Build history of the part. All positions in model axes, mm. Face numbers are marked on the shaded views. A direction names the side the tool comes from. Round coordinates to 2 decimals unless told otherwise and drop trailing zeros. Loops run counter-clockwise (first coordinate to the right, second up) from the corner with the lowest first, then second, coordinate; pieces in that order, holes last. Notation, with made-up numbers: M -28,-37 L -22,-37 A20 cw -22,-29 Z; hole C 69,35 d5. An arc over 180 degrees is marked long. Write each question's results on one line, items separated by ' | '. Start each with the question number.
```python
from build123d import *

# Parameters (mm, degrees)
BOSS_EXTRUDE1_DEPTH = 1.366666667
BOSS_EXTRUDE2_DEPTH = 8.2
FILLET1_R           = 0.5


with BuildPart() as part:
    # Sketch1 → Boss-Extrude1 (new body)
    with BuildSketch(Plane.XY):
        with BuildLine():
            Line((-33.5, 20), (-33.5, -20))
            ThreePointArc((-33.5, -20), (0, -17.434472888), (33.5, -20))
            Line((33.5, -20), (33.5, 20))
            Line((33.5, 20), (-33.5, 20))
        make_face()
    extrude(amount=BOSS_EXTRUDE1_DEPTH)

    # Sketch2 → Boss-Extrude2 (add)
    with BuildSketch(Plane.XY.offset(1.366666667)):
        with BuildLine():
            Line((32.5, -15), (-32.5, -15))
            Line((-32.5, -15), (-32.5, 15))
            ThreePointArc((-32.5, 15), (0, 17.727407049), (32.5, 15))
            Line((32.5, 15), (32.5, -15))
        make_face()
    extrude(amount=BOSS_EXTRUDE2_DEPTH)

    # Fillet1
    fillet1_edges = [part.edges().sort_by_distance(p)[0] for p in [
        (33.5, 0, 1.366666667),
        (-33.5, 0, 1.366666667),
    ]]
    fillet(fillet1_edges, radius=FILLET1_R)


solid = part.part
```
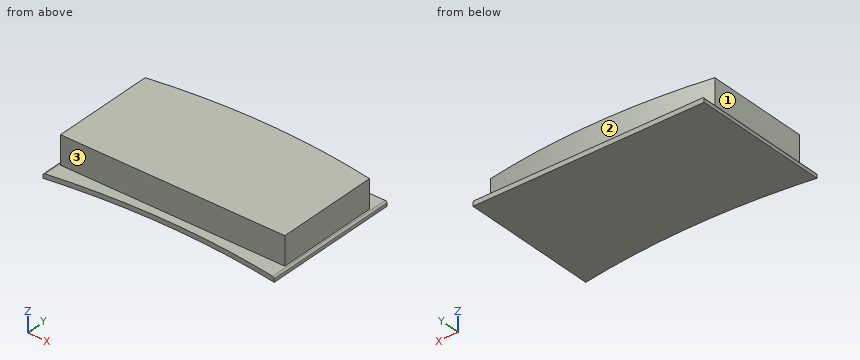
Item 1: Saw through at C-C, the plane z = 7.5. Give the cut face in (x, y).
Item 2: Saw through at B-B, the plane y = 10. Give the cut face in (x, z).
Item 3: Drill centre lines: line 1 along X through (y, z) = (-8, 3.75); line 2 along Z through (x, y) = (-9, -17); line 3 along Y through (x, z) = (-10, 8.75). Where is each one in solid material? Low to high. Write a range as [from, to].
Item 4: Tool access for the marked faces 1, 2 and 3: list every direction of +Z, -Z, +X, -X, +Y, -Y with a clear straight run to the whole face (end or side of a thin tool).
Item 5: Drop flat-ended pins along their axis: pin 1 (4 mm diameter, centred on x = 25, z = 6.5, fed in from +Y); pin 2 (4 mm diameter, centred on y = -5.5, z = 3.5, fed in from +X); pin 3 (4 mm diameter, centred on x = 1, z = 5.5, fed in from -Y). Give the stop position or say it passes through.
Item 6: Saw through at D-D, the plane x = -9. Give the cut face in (y, z), then the cut area to 3 significant figures.
Item 7: Saw through at A-A, the plane x = -25. Give the cut face in (y, z).
Working result:
1) outline: M -32.5,-15 L 32.5,-15 L 32.5,15 A195 ccw -32.5,15 Z
2) outline: M -33.5,0 L 33.5,0 L 33.5,0.87 A0.5 ccw 33,1.37 L 32.5,1.37 L 32.5,9.57 L -32.5,9.57 L -32.5,1.37 L -33,1.37 A0.5 ccw -33.5,0.87 Z
3) line 1: x = [-32.5, 32.5] | line 2: z = [0, 1.37] | line 3: y = [-15, 17.47]
4) face 1: +Z, -X, +Y, -Y | face 2: +Z, +Y | face 3: +Z, +X, -X, -Y
5) pin 1: stops at y = 16.37 | pin 2: stops at x = 32.5 | pin 3: stops at y = -15
6) outline: M -17.62,0 L 20,0 L 20,1.37 L 17.52,1.37 L 17.52,9.57 L -15,9.57 L -15,1.37 L -17.62,1.37 Z | area: 318 mm²
7) outline: M -18.86,0 L 20,0 L 20,1.37 L 16.12,1.37 L 16.12,9.57 L -15,9.57 L -15,1.37 L -18.86,1.37 Z
